Could you check a few things on this drawing? It's one solid part, dimensions in mm from its lowest x, y, z. Coordinates: 2 decimals unless noted, no trailing zeros. Order: outer loops, then holes, each group sorted by start corner. A loop starts at its lowest first (then second) coordinate and runs counter-clockwise, first axis right, second up.
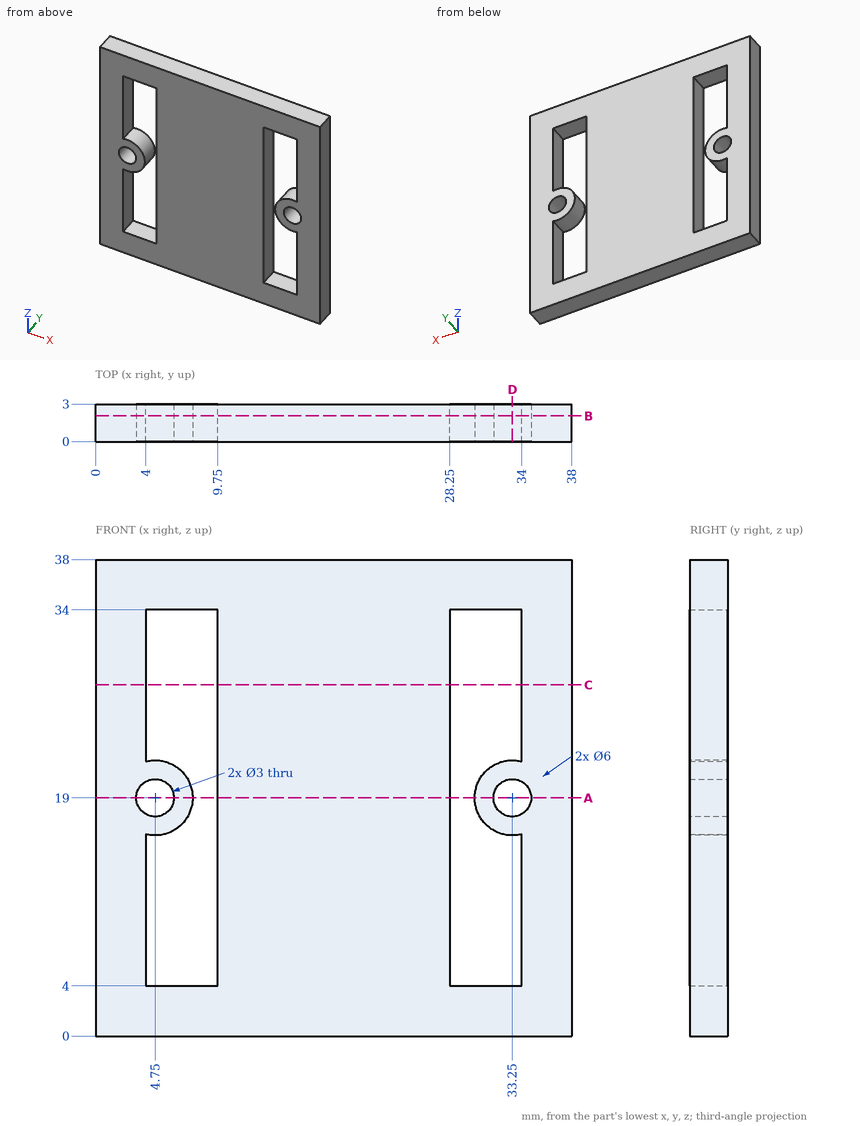
1. Imagine slicing it at A-A on z = 19. Please give me the cut outline in (x, y).
Completed:
outline: (0, 0) - (3.25, 0) - (3.25, 3) - (0, 3) - close; (6.25, 0) - (7.75, 0) - (7.75, 3) - (6.25, 3) - close; (9.75, 0) - (28.25, 0) - (28.25, 3) - (9.75, 3) - close; (30.25, 0) - (31.75, 0) - (31.75, 3) - (30.25, 3) - close; (34.75, 0) - (38, 0) - (38, 3) - (34.75, 3) - close
2. Imagine slicing it at C-C on z = 28. Please give me the cut outline in (x, y).
Completed:
outline: (0, 0) - (4, 0) - (4, 3) - (0, 3) - close; (9.75, 0) - (28.25, 0) - (28.25, 3) - (9.75, 3) - close; (34, 0) - (38, 0) - (38, 3) - (34, 3) - close
3. Please list where these lines run through material, in increasing order: probe 1 along X at (y, z) = (2.7, 5); probe 2 along Z at (x, y) = (32, 0.4); probe 3 along Z at (x, y) = (33.5, 2.35).
Completed:
probe 1: x = 0 to 4, 9.75 to 28.25, 34 to 38
probe 2: z = 0 to 4, 16.27 to 18.17, 19.83 to 21.73, 34 to 38
probe 3: z = 0 to 4, 16.01 to 17.52, 20.48 to 21.99, 34 to 38
4. Imagine slicing it at B-B on y = 2.05. Please give me the cut outline in (x, z).
Completed:
outline: (0, 0) - (38, 0) - (38, 38) - (0, 38) - close; hole circle Ø3 at (4.75, 19); hole (4, 4) - (9.75, 4) - (9.75, 34) - (4, 34) - (4, 21.9) arc R3 cw (long way) to (4, 16.1) - close; hole (28.25, 4) - (34, 4) - (34, 16.1) arc R3 cw (long way) to (34, 21.9) - (34, 34) - (28.25, 34) - close; hole circle Ø3 at (33.25, 19)
5. Imagine slicing it at D-D on x = 33.25. Please give me the cut outline in (y, z).
Completed:
outline: (0, 0) - (3, 0) - (3, 4) - (0, 4) - close; (0, 16) - (3, 16) - (3, 17.5) - (0, 17.5) - close; (0, 20.5) - (3, 20.5) - (3, 22) - (0, 22) - close; (0, 34) - (3, 34) - (3, 38) - (0, 38) - close
